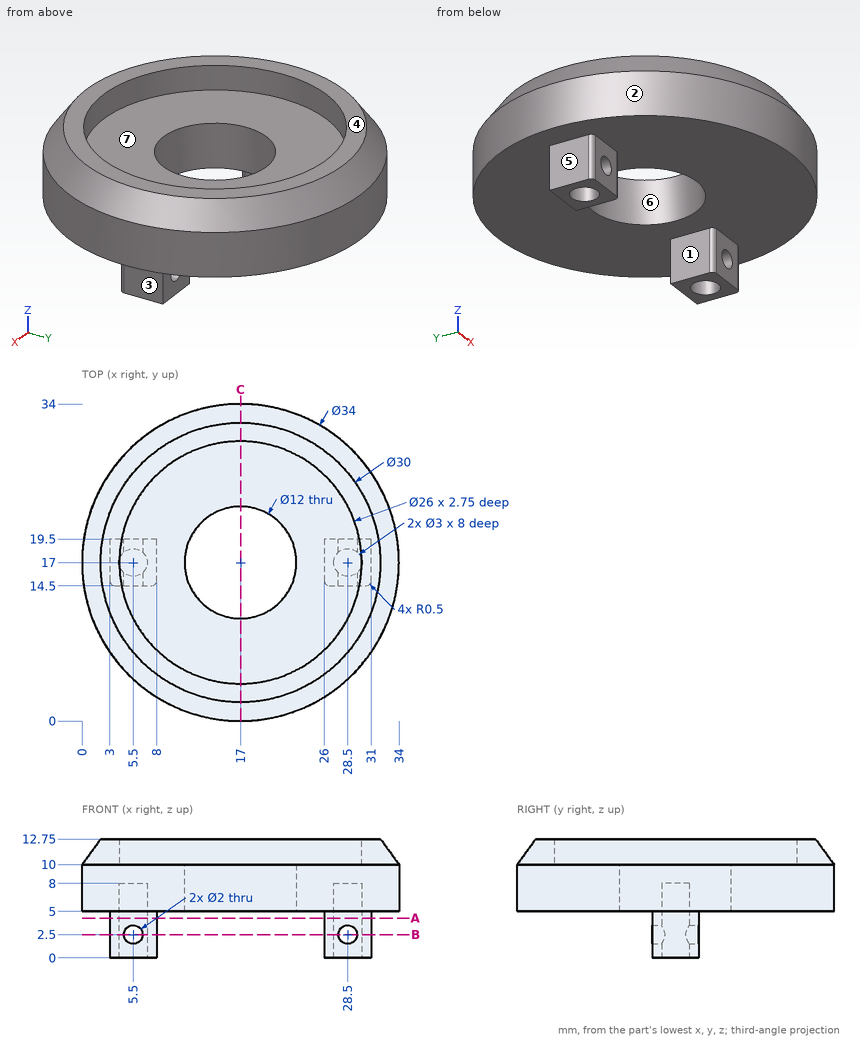
Answer from the drawing. Dimensions are ordinates in mm from the lowest x, y and z of the part. A direction names the side the tool comes from. Round coordinates to 2 decimals unless told otherwise and drop trailing zeros. Loops run counter-clockwise (first coordinate to the right, second up) from the corner with the lowest first, then second, coordinate; pieces in that order, holes last.
Q1. Each of these flat-tipped pins is pushed along its axis until it touches: pin 1 (6 mm diameter, centred on x = 11.5, z = 4, fed in from -Y); pin 2 (2.5 mm diameter, centred on x = 28.5, z = 2.5, fed in from -Y); pin 3 (2.5 mm diameter, centred on x = 5.5, y = 17, fed in from +Z). Where does it stop, or does it pass through?
Q2. Determine the mould class of the marked faces 1, 2, 3 and 4 for opening direction X: released by +X, released by -X, zero draft, split by the parting line, or undercut.
Q3. Section A-A on z = 4.25 is taken. Write down the section's boundary in (x, y), and give its area (3 significant figures).
Q4. Section B-B on z = 2.5 is taken. Write down the section's boundary in (x, y), and give its area (3 significant figures).
Q5. Section C-C on x = 17 is taken. Write down the section's boundary in (y, z), and give its area (4 significant figures).
Q6. Which of the six approach directions +Z, -Z, +X, -X, +Y, -Y give full straight-line access (tool end or side, diameter ignored) to the marked faces 5, 6 and 7?
Q7. Consider probe 1 along Z at (x, y) = (5.5, 15.4); probe 2 along Z at (x, y) = (22, 8); probe 3 along Y at (x, z) = (12, 7). Determine where each line is inside the solid, lowest interval first.
Output:
1. pin 1: stops at y = 0.21
1. pin 2: stops at y = 14.5
1. pin 3: stops at z = 10
2. face 1: undercut
2. face 2: split by the parting line
2. face 3: released by +X
2. face 4: zero draft
3. outline: (3, 15) arc R0.5 ccw to (3.5, 14.5) - (7.5, 14.5) arc R0.5 ccw to (8, 15) - (8, 19.5) - (3, 19.5) - close; (26, 15) arc R0.5 ccw to (26.5, 14.5) - (30.5, 14.5) arc R0.5 ccw to (31, 15) - (31, 19.5) - (26, 19.5) - close; hole circle Ø3 at (5.5, 17); hole circle Ø3 at (28.5, 17)
3. area: 35.6 mm2
4. outline: (3, 15) arc R0.5 ccw to (3.5, 14.5) - (4.5, 14.5) - (4.5, 15.88) arc R1.5 cw to (4.5, 18.12) - (4.5, 19.5) - (3, 19.5) - close; (6.5, 14.5) - (7.5, 14.5) arc R0.5 ccw to (8, 15) - (8, 19.5) - (6.5, 19.5) - (6.5, 18.12) arc R1.5 cw to (6.5, 15.88) - close; (26, 15) arc R0.5 ccw to (26.5, 14.5) - (27.5, 14.5) - (27.5, 15.88) arc R1.5 cw to (27.5, 18.12) - (27.5, 19.5) - (26, 19.5) - close; (29.5, 14.5) - (30.5, 14.5) arc R0.5 ccw to (31, 15) - (31, 19.5) - (29.5, 19.5) - (29.5, 18.12) arc R1.5 cw to (29.5, 15.88) - close
4. area: 26.7 mm2
5. outline: (0, 5) - (11, 5) - (11, 10) - (4, 10) - (4, 12.75) - (2, 12.75) - (0, 10) - close; (23, 5) - (34, 5) - (34, 10) - (32, 12.75) - (30, 12.75) - (30, 10) - (23, 10) - close
5. area: 126.5 mm2
6. face 5: -Z, -X, +Y, -Y
6. face 6: +Z, -Z
6. face 7: +Z
7. probe 1: z = 0 to 1.5, 3.5 to 10
7. probe 2: z = 5 to 10
7. probe 3: y = 0.75 to 13.68, 20.32 to 33.25
